Design review of the part built by this model. Coordinates are the model's own, in mm. Face numbers are marked on the shaded views. Give positions to 0.01 mm unless a question says otherwise; leave off trailing zeros. Loops run counter-clockwise (first coordinate to the right, second up) from the corner with the lowest first, then second, coordinate; pieces in that order, holes last. Notation, with made-up numbers: M 8,21 L 41,21 A24 cw 41,58 Z; hole C 75,-2.5 d6. An arc over 180 degrees is marked long. Use a Markdown table: item, result. Add a question column.
(1) Add section A-A, the plane z = -130.5. Give the boundary of the cut face in (x, y), then the cut area to 3 significant figures.
(2) Draft analysis for pull direction X (two halves, no side actions). For the marked faces 1, 2 and 3, state which applies: pulls with the +X half, pulls with the -X half, needs draft (parallel to the pull), parting line crosses it, or undercut.
(3) Insertion check: pin 1 Ø1 at (x, y) = (18, 20.5) entering from -Z; pin 2 Ø5 at (x, y) = (-6, -23) entering from +Z; pin 3 Ø16.5 at (y, z) = (20, -181) entering from +X. Each pin has a flat end and moves straight along its axis. Give the tip position at first contact, or say it passes through.
(4) Add section B-B, the plane z = -194.5. Give the boundary of the cut face in (x, y).
(5) For probe 1 along X at (y, z) = (-14, -196.5); probe 2 along X at (y, z) = (-9, -203.5); probe 3 along X at (y, z) = (0.5, -164.5), list the stretches that pass through material, from the lowest coordinate up.
```python
from build123d import *

# Parameters (mm, degrees)
BOSS_EXTRUDE1_DEPTH = 2.5
CIRPATTERN2_COUNT   = 3


with BuildPart() as part:
    # Sketch1 → Revolve1 (revolve)
    with BuildSketch(Plane(origin=(0, 0, 0), x_dir=(0, 0, -1), z_dir=(1, 0, 0)), mode=Mode.PRIVATE) as revolve1_sk:
        with BuildLine():
            Line((225, 0), (225, 7.5))
            Line((225, 7.5), (70.12061166, 7.5))
            add(Edge.make_bspline(
                [(70.12061166, 7.5), (56.641182796, 25.980733589), (33.840993592, 41.275), (0, 41.275)],
                knots=[0.117191472, 0.117191472, 0.117191472, 0.117191472, 1, 1, 1, 1], degree=3))
            add(Edge.make_bspline(
                [(-75, 0), (-62.5, 21.650635095), (-38.333333333, 41.275), (0, 41.275)],
                knots=[0, 0, 0, 0, 1, 1, 1, 1], degree=3))
            Line((-75, 0), (225, 0))
        make_face()
    revolve(revolve1_sk.sketch.rotate(Axis((0, 0, 75), (0, 0, -1)), 180), axis=Axis((0, 0, 75), (0, 0, -1)))

    # Sketch2 → Boss-Extrude1 (add, symmetric)
    with BuildSketch(Plane(origin=(0, 0, 0), x_dir=(0, 0, -1), z_dir=(1, 0, 0))):
        Polygon((185, 40), (141.698729811, 15), (52.71703536, 15), (52.71703536, 0), (210, 0), (225, 15), (221.464466094, 36.464466094), align=None)
    boss_extrude1 = extrude(amount=BOSS_EXTRUDE1_DEPTH, both=True)

    # CirPattern2: Boss-Extrude1 ×3 about axis
    cirpattern2_axis = Axis((0, 0, 0), (0, 0, 1))
    for i in range(1, CIRPATTERN2_COUNT):
        add(boss_extrude1.rotate(cirpattern2_axis, i * 360 / CIRPATTERN2_COUNT))


solid = part.part
```
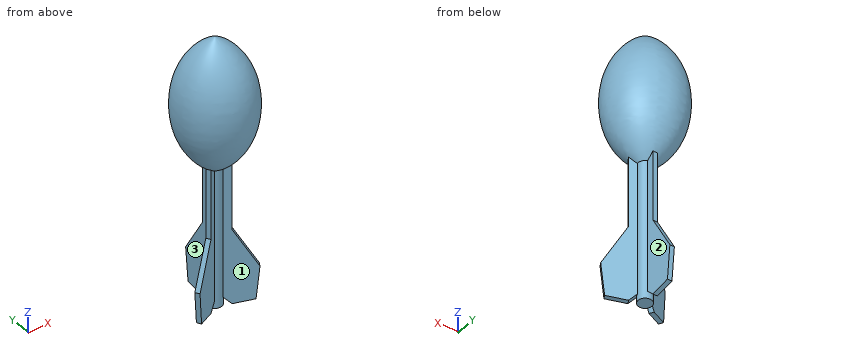
Established:
| question | item | result |
|---|---|---|
| 1 | outline | M -14.24,-5.33 L -11.74,-9.67 L -4.87,-5.7 A7.5 ccw 4.87,-5.7 L 11.74,-9.67 L 14.24,-5.33 L 7.37,-1.37 A7.5 ccw 2.5,7.07 L 2.5,15 L -2.5,15 L -2.5,7.07 A7.5 ccw -7.37,-1.37 Z |
| 1 | area | 291 mm^2 |
| 2 | face 1 | undercut |
| 2 | face 2 | pulls with the +X half |
| 2 | face 3 | pulls with the -X half |
| 3 | pin 1 | z = -50.24 |
| 3 | pin 2 | z = 57.44 |
| 3 | pin 3 | x = 2.5 |
| 4 | outline | M -35.09,-17.37 L -32.59,-21.7 L -4.87,-5.7 A7.5 ccw 4.87,-5.7 L 32.59,-21.7 L 35.09,-17.37 L 7.37,-1.37 A7.5 ccw 2.5,7.07 L 2.5,39.08 L -2.5,39.08 L -2.5,7.07 A7.5 ccw -7.37,-1.37 Z |
| 5 | probe 1 | -29.25 to -19.25, 19.25 to 29.25 |
| 5 | probe 2 | -20.59 to -10.59, 10.59 to 20.59 |
| 5 | probe 3 | -7.48 to 7.48 |
